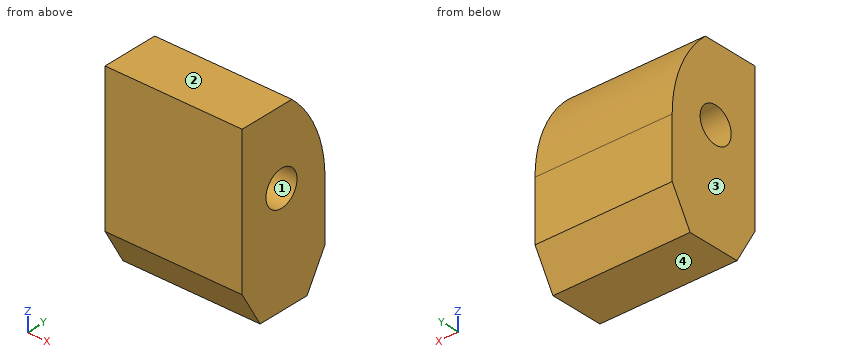
```python
from build123d import *

# Parameters (mm, degrees)
SKETCH1_R           = 7.5
BOSS_EXTRUDE1_DEPTH = 29


with BuildPart() as part:
    # Sketch1 → Boss-Extrude1 (new, symmetric)
    with BuildSketch(Plane(origin=(0, 0, 0), x_dir=(0, 0, -1), z_dir=(1, 0, 0))):
        with BuildLine():
            Line((-31, 5), (-31, -19))
            Line((-31, -19), (31, -19))
            Line((31, -19), (46, -10.339745962))
            Line((46, -10.339745962), (46, 12.339745962))
            Line((46, 12.339745962), (31, 21))
            Line((31, 21), (5.66060556, 21))
            ThreePointArc((5.66060556, 21), (-14.33939444, 16.82575695), (-31, 5))
        make_face()
        with Locations(Location((0, 0, 0), (0, 0, 180))):
            Circle(SKETCH1_R, mode=Mode.SUBTRACT)
    extrude(amount=BOSS_EXTRUDE1_DEPTH, both=True)


solid = part.part
```
Input: part model. Units: mm. Frame: model coordinates. Face numbers are marked on the shaded views. Round coordinates to 2 decimals unless told otherwise and drop trailing zeros. Loops run counter-clockwise (first coordinate to the right, second up) from the corner with the lowest first, then second, coordinate; pieces in that order, holes last.
1) Section query C-C on z = -2. Return the cut outline in (x, y).
Ans:
outline: (-29, -19) - (29, -19) - (29, -7.23) - (-29, -7.23) - close; (-29, 7.23) - (29, 7.23) - (29, 20.87) - (-29, 20.87) - close
2) Pin query (flat end, axial travel): pin 1 (13.5 mm diameter, centred on y = 0, z = 0, fed in from +X); pin 2 (5 mm diameter, centred on y = 16, z = 21, fed in from -X); pin 3 (1.5 mm diameter, centred on x = 22.5, z = -37.5, fed in from +Y); pin 4 (1 mm diameter, centred on x = -18.5, y = -14, fed in from -Z). Return the tip coordinate at first contact, or that it passes through.
Ans:
pin 1: passes through
pin 2: stops at x = -29
pin 3: stops at y = 17.68
pin 4: stops at z = -40.53
3) Pull-direction query (Z, two-part tool) for the marked faces 1, 2, 3 and 4; classes: released by +Z, released by -Z, zero draft, split by the parting line, or undercut.
Ans:
face 1: undercut
face 2: released by +Z
face 3: zero draft
face 4: released by -Z
4) Section query A-A on y = 0. Return the cut outline in (x, z), plus the area to 3 significant figures.
Ans:
outline: (-29, -46) - (29, -46) - (29, -7.5) - (-29, -7.5) - close; (-29, 7.5) - (29, 7.5) - (29, 31) - (-29, 31) - close
area: 3,600 mm2
5) Section query B-B on x = -7. Return the cut outline in (y, z).
Ans:
outline: (-19, -31) - (-10.34, -46) - (12.34, -46) - (21, -31) - (21, -5.66) arc R50 ccw to (5, 31) - (-19, 31) - close; hole circle Ø15 at (0, 0)
6) Section query D-D on y = 17. Return the cut outline in (x, z).
Ans:
outline: (-29, -37.93) - (29, -37.93) - (29, 13.94) - (-29, 13.94) - close
7) Material intervals for line 1 (Z direction, x = -12, y = 0.5); line 2 (Z direction, x = 23, y = -1); line 3 (Y direction, x = -6.5, z = 0), sorted ascending.
Ans:
line 1: z = -46 to -7.48, 7.48 to 31
line 2: z = -46 to -7.43, 7.43 to 31
line 3: y = -19 to -7.5, 7.5 to 20.68
